The listing builds one solid part. Answer for the finished solid, in the listing's coordinates (mm). Coordinates: 2 decimals unless noted, no trailing zeros. Write each loop counter-clockwise with the first axis right and the second up, starting at its lowest first coordinate (ties: lowest second). Pieces come first, ordered by that corner, then holes.
from build123d import *

# Parameters (mm, degrees)
F0_W     = 50.8
F0_H     = 30.48
F1_DEPTH = 7.112
F2_R     = 11.176
F3_DEPTH = 25.4
F4_R     = 2.54


with BuildPart() as f1:
    # F0 (on Top) → F1 (new body)
    with BuildSketch(Plane.XY):
        Rectangle(F0_W, F0_H)
        with BuildLine():
            ThreePointArc((25.4, -15.24), (40.64, 0), (25.4, 15.24))
            Line((25.4, 15.24), (25.4, -15.24))
        make_face()
        with BuildLine():
            Line((-25.4, -15.24), (-25.4, 15.24))
            ThreePointArc((-25.4, 15.24), (-40.64, 0), (-25.4, -15.24))
        make_face()
    extrude(amount=F1_DEPTH)

    # F2 (on face) → F3 (cut)
    with BuildSketch(Plane.XY.offset(7.112)):
        Circle(F2_R)
        with Locations((-25.4, 0)):
            Circle(F2_R)
        with Locations((25.4, 0)):
            Circle(F2_R)
    extrude(amount=-F3_DEPTH, mode=Mode.SUBTRACT)

    # F4
    f4_edges = [f1.edges().sort_by_distance(p)[0] for p in [
        (0, 15.24, 0),
        (-40.64, 0, 0),
        (0, -15.24, 0),
        (40.64, 0, 0),
        (40.64, 0, 7.112),
        (0, 15.24, 7.112),
        (-40.64, 0, 7.112),
        (0, -15.24, 7.112),
    ]]
    fillet(f4_edges, radius=F4_R)


solid = f1.part
1. Section A-A on y = 0 is taken. Give the vertices of the cut face in (x, z).
Results found:
outline: (-40.64, 2.54) arc R2.54 ccw to (-38.1, 0) - (-36.58, 0) - (-36.58, 7.11) - (-38.1, 7.11) arc R2.54 ccw to (-40.64, 4.57) - close; (-14.22, 0) - (-11.18, 0) - (-11.18, 7.11) - (-14.22, 7.11) - close; (11.18, 0) - (14.22, 0) - (14.22, 7.11) - (11.18, 7.11) - close; (36.58, 0) - (38.1, 0) arc R2.54 ccw to (40.64, 2.54) - (40.64, 4.57) arc R2.54 ccw to (38.1, 7.11) - (36.58, 7.11) - close
2. For a pull along Y with two mould halves and no side action, classify faces 1 (the cylindrical face through (-8.87, -6.8, 3.61)), 2 (the flat face through (-11.5, 0.1, 7.112)), 3 (the cylindrical face through (-0.356, -14.476, 0.724)) as pulls with the +Y half, pulls with the -Y half, needs draft (parallel to the pull), parting line crosses it, or undercut.
Results found:
face 1: undercut
face 2: needs draft
face 3: pulls with the -Y half
3. Flat-ended cylindrical pins translate along their axes: P1, Ø18, axis at x = 25.4, y = 0, coming from the +Z side; P2, Ø1.5, axis at y = -2, z = 2.5, coming from the -X side. Find the tip coordinate at first contact, or state that the pin passes through.
Results found:
P1: passes through
P2: stops at x = -40.59
4. Section D-D on x = -16.5 is taken. Give the vertices of the cut face in (y, z).
Results found:
outline: (-15.24, 2.54) arc R2.54 ccw to (-12.7, 0) - (-6.76, 0) - (-6.76, 7.11) - (-12.7, 7.11) arc R2.54 ccw to (-15.24, 4.57) - close; (6.76, 0) - (12.7, 0) arc R2.54 ccw to (15.24, 2.54) - (15.24, 4.57) arc R2.54 ccw to (12.7, 7.11) - (6.76, 7.11) - close
5. Section B-B on x = 0 is taken. Give the vertices of the cut face in (y, z).
Results found:
outline: (-15.24, 2.54) arc R2.54 ccw to (-12.7, 0) - (-11.18, 0) - (-11.18, 7.11) - (-12.7, 7.11) arc R2.54 ccw to (-15.24, 4.57) - close; (11.18, 0) - (12.7, 0) arc R2.54 ccw to (15.24, 2.54) - (15.24, 4.57) arc R2.54 ccw to (12.7, 7.11) - (11.18, 7.11) - close
6. Section C-C on z = 6 is taken. Give the vertices of the cut face in (x, y), then the cut area to 3 significant figures.
Results found:
outline: (-25.4, -14.8) - (25.4, -14.8) arc R14.8 ccw to (25.4, 14.8) - (-25.4, 14.8) arc R14.8 ccw to start; hole circle Ø22.35 at (-25.4, 0); hole circle Ø22.35 at (0, 0); hole circle Ø22.35 at (25.4, 0)
area: 1,010 mm2
7. Find the intervals of material crossed by L1, parallel to Y at x = 0, z = 2.25; L2, parallel to X at y = 8.5, z = 4; L3, parallel to X at y = -9, z = 0.75, in increasing order.
Results found:
L1: y = -15.22 to -11.18, 11.18 to 15.22
L2: x = -38.05 to -32.66, -18.14 to -7.26, 7.26 to 18.14, 32.66 to 38.05
L3: x = -36.77 to -32.03, -18.77 to -6.63, 6.63 to 18.77, 32.03 to 36.77
